The figure shows three views and two pictorial views of one solid part (mm, origin at its lowest corner). Answer the questions. A direction names the side the tool comes from. Give positions to 0.01 mm unless a question says otherwise; leave off trailing zeros. Write each loop counter-clockwise with the first axis right and the second up, starting at its lowest first coordinate (ties: lowest second). Pieces come first, ordered by that corner, then holes. Notation, with made-up numbers: (62.25, 82) - (111.25, 82) arc R27 cw to (111.25, 121) - close; hole circle Ø11 at (32.25, 28.25). An arc over 180 degrees is marked (long way). One line per question, with ' | ' between items. Start each with the question number.
1. A cutting plane is placed at A-A (z = 18.5). State how many separate pieces and enclosed holes the cut face has.
2. A cutting plane is placed at C-C (x = 9.25). Determine the outline of the cut face in (y, z), then the cut area to 3 significant figures.
3. For the marked faces 1, 2, 3, 4 and 5, determine the directions among +Z, -Z, +X, -X, +Y, -Y from which every point of the face is accessible in a straight line to the end or side of a thin tool.
4. Given P1, Ø1.7, axis at y = 3, z = 28.5, coming from the +X side; P2, Ø10, axis at x = 14.5, z = 13, coming from the +Y side; P3, Ø2.5, axis at y = 3.5, z = 9, coming from the -X side; P4, Ø1.8, axis at x = 27, y = 3.5, coming from the -Z side, each flat-ended and moving along its own axis, determine where each tip first touches the part or whether it passes through.
5. Find the intervals of material crossed by L1, parallel to Z at x = 24.25, y = 3.95; L2, parallel to Z at x = 16, y = 1.8; L3, parallel to X at y = 5.15, z = 8.5, in increasing order. Write a range as from..to.
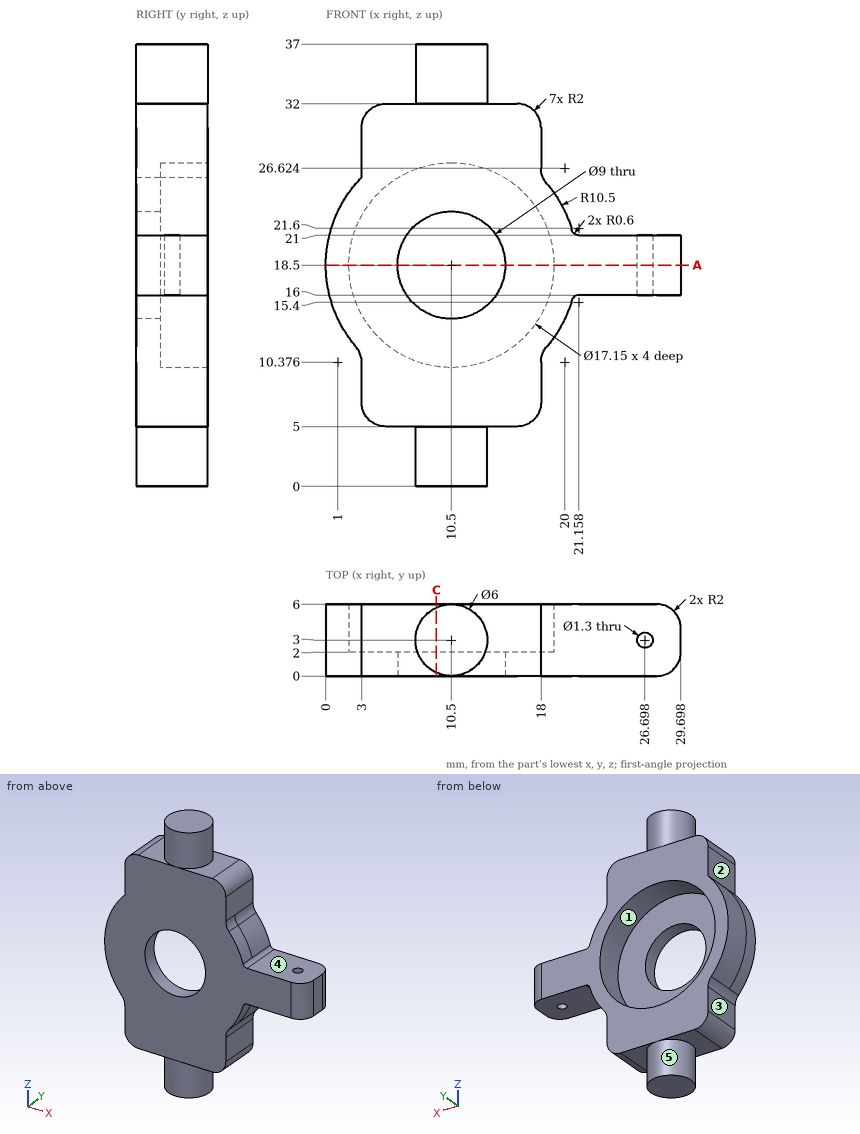
Determined:
1) separate pieces: 2 | enclosed holes: 1
2) outline: (0, 5) - (0.27, 5) - (0.27, 0) - (5.73, 0) - (5.73, 5) - (6, 5) - (6, 10.02) - (2, 10.02) - (2, 14.18) - (0, 14.18) - close; (0, 22.82) - (2, 22.82) - (2, 26.98) - (6, 26.98) - (6, 32) - (5.73, 32) - (5.73, 37) - (0.27, 37) - (0.27, 32) - (0, 32) - close | area: 131 mm2
3) face 1: +Y | face 2: +Z, -X, +Y, -Y | face 3: -Z, -X, +Y, -Y | face 4: +Z, +X, +Y, -Y | face 5: -Z
4) P1: x = 18 | P2: y = 6 | P3: x = 3 | P4: z = 16
5) L1: 16..21 | L2: 5..32 | L3: 3..18
